from build123d import *

# Parameters (mm, degrees)
SKETCH1_W           = 40
SKETCH1_H           = 50
BOSS_EXTRUDE1_DEPTH = 5
SKETCH4_W           = 15
SKETCH4_H           = 5
SKETCH4_W_2         = 5
BOSS_EXTRUDE5_DEPTH = 10
CUT_EXTRUDE2_DEPTH  = 4
BOSS_EXTRUDE7_START = 3
BOSS_EXTRUDE7_DEPTH = 3
SKETCH9_W           = 5
SKETCH9_H           = 5
BOSS_EXTRUDE8_DEPTH = 5
SKETCH10_R          = 1.5
CUT_EXTRUDE3_DEPTH  = 5


with BuildPart() as part:
    # Sketch1 → Boss-Extrude1 (new body)
    with BuildSketch(Plane(origin=(0, 0, 0), x_dir=(1, 0, 0), z_dir=(0, 1, 0))):
        Rectangle(SKETCH1_W, SKETCH1_H)
    extrude(amount=BOSS_EXTRUDE1_DEPTH)

    # Sketch4 → Boss-Extrude5 (add)
    with BuildSketch(Plane(origin=(0, 5, 0), x_dir=(1, 0, 0), z_dir=(0, 1, 0))):
        Polygon((20, -25), (20, 25), (16, 25), (16, -20), (-7, -20), (-7, -25), align=None)
        with Locations((0.5, 22.5)):
            Rectangle(SKETCH4_W, SKETCH4_H)
        with Locations((-17.5, 22.5)):
            Rectangle(SKETCH4_W_2, SKETCH4_H)
        with Locations((-9.5, -22.5)):
            Rectangle(SKETCH4_W_2, SKETCH4_H)
    extrude(amount=BOSS_EXTRUDE5_DEPTH)

    # Sketch7 → Cut-Extrude2 (cut)
    with BuildSketch(Plane(origin=(20, 0, 0), x_dir=(0, 0, -1), z_dir=(1, 0, 0))):
        with BuildLine():
            Line((-1, 15), (21, 15))
            ThreePointArc((21, 15), (10, 4), (-1, 15))
        make_face()
    extrude(amount=-CUT_EXTRUDE2_DEPTH, mode=Mode.SUBTRACT)

    # Sketch8 → Boss-Extrude7 (add)
    with BuildSketch(Plane(origin=(20, 0, 0), x_dir=(0, 0, -1), z_dir=(1, 0, 0)).offset(BOSS_EXTRUDE7_START)):
        with BuildLine():
            Line((-1, 15), (-4, 15))
            Line((-4, 15), (-4, 0))
            Line((-4, 0), (24, 0))
            Line((24, 0), (24, 15))
            Line((24, 15), (21, 15))
            ThreePointArc((21, 15), (10, 4), (-1, 15))
        make_face()
    extrude(amount=-BOSS_EXTRUDE7_DEPTH)

    # Sketch9 → Boss-Extrude8 (add)
    with BuildSketch(Plane(origin=(0, 0, -25), x_dir=(-1, 0, 0), z_dir=(0, 0, -1))):
        with Locations((0, 12.5)):
            Rectangle(SKETCH9_W, SKETCH9_H)
    extrude(amount=BOSS_EXTRUDE8_DEPTH)

    # Sketch10 → Cut-Extrude3 (cut)
    with BuildSketch(Plane.XZ.offset(-10)):
        with Locations(Location((0, -27.5, 0), (0, 0, 270))):
            Circle(SKETCH10_R)
    extrude(amount=-CUT_EXTRUDE3_DEPTH, mode=Mode.SUBTRACT)


solid = part.part
Source: CAD feature listing. Evaluate the final solid. Frame: model axes, mm. A direction names the side the tool comes from. Coordinates: 2 decimals unless noted, no trailing zeros. Order: outer loops, then holes, each group sorted by start corner. A loop starts at its lowest first (then second) coordinate and runs counter-clockwise, first axis right, second up.
Item 1: Pull-direction query (X, two-part tool) for faces 1 (the face through (0, 12, -26)), 2 (the face through (2.5, 12, -27)), 3 (the face through (20, 15, -23)); classes: pulls with the +X half, pulls with the -X half, needs draft (parallel to the pull), parting line crosses it, or undercut.
Output values:
face 1: undercut
face 2: pulls with the +X half
face 3: needs draft
Item 2: Cut plane A-A (y = 13.5). Return loops of the section in (x, z).
Output values:
outline: (-20, -25) - (-15, -25) - (-15, -20) - (-20, -20) - close; (-12, 20) - (16, 20) - (16, 0.9) - (23, 0.9) - (23, 4) - (20, 4) - (20, 25) - (-12, 25) - close; (-7, -25) - (-2.5, -25) - (-2.5, -30) - (2.5, -30) - (2.5, -25) - (8, -25) - (8, -20) - (-7, -20) - close; (16, -25) - (20, -25) - (20, -24) - (23, -24) - (23, -20.9) - (16, -20.9) - close; hole circle Ø3 at (0, -27.5)
Item 3: Cut plane D-D (y = 5.75). Return loops of the section in (x, z), plus the area to 3 significant figures.
Output values:
outline: (-20, -25) - (-15, -25) - (-15, -20) - (-20, -20) - close; (-12, 20) - (16, 20) - (16, -4.05) - (23, -4.05) - (23, 4) - (20, 4) - (20, 25) - (-12, 25) - close; (-7, -25) - (8, -25) - (8, -20) - (-7, -20) - close; (16, -25) - (20, -25) - (20, -24) - (23, -24) - (23, -15.95) - (16, -15.95) - close
area: 441 mm2
Item 4: Cut plane C-C (z = -27.5). Return loops of the section in (x, y).
Output values:
outline: (-2.5, 10) - (-1.5, 10) - (-1.5, 15) - (-2.5, 15) - close; (1.5, 10) - (2.5, 10) - (2.5, 15) - (1.5, 15) - close
Item 5: Material intervals for line 1 (X direction, y = 11.1, z = -27.5); line 2 (Z direction, x = 5.5, y = 1.25); line 3 (Y direction, x = 5, z = 8), sorted ascending.
Output values:
line 1: x = -2.5 to -1.5, 1.5 to 2.5
line 2: z = -25 to 25
line 3: y = 0 to 5
Item 6: Set-up query: faces 4 (the face through (0, 10, -20)), 5 (the face through (16, 10, 10)), 6 (the face through (22, 7, -24)). Return all of +Z, -Z, +X, -X, +Y, -Y with unobstructed straight access to the full face (end or side cutting, diameter ignored); none if empty.
Output values:
face 4: -X, +Y
face 5: -Z, -X, +Y
face 6: -Z, +X, +Y, -Y
Item 7: Cut plane B-B (x = 0). Return loops of the section in (y, z), plus the area to 3 significant figures.
Output values:
outline: (0, -25) - (10, -25) - (10, -26) - (15, -26) - (15, -20) - (5, -20) - (5, 20) - (15, 20) - (15, 25) - (0, 25) - close; (10, -30) - (15, -30) - (15, -29) - (10, -29) - close
area: 360 mm2
Item 8: First-contact query: P1, Ø0.9, axis at x = 21.5, y = 7.5, coming from the +Z side; P2, Ø5, axis at x = -7.5, y = 5.5, coming from the -Z side; P3, Ø0.5, axis at y = 9.5, z = -24.5, coming from the +X side. Flat tips, straight axial feed; report the tip coordinate or a pass-through.
Output values:
P1: stops at z = 4
P2: stops at z = -25
P3: stops at x = 20
